Verification items for the finished model (mm, model axes). A direction names the side the tool comes from. Give positions to 0.01 mm unless a question says otherwise; leave off trailing zeros. Order: outer loops, then holes, each group sorted by start corner. A loop starts at its lowest first (then second) coordinate and runs counter-clockwise, first axis right, second up. Notation, with made-up numbers: (39.5, 17.5) - (46.5, 17.5) arc R31 ccw to (46.5, 47.5) - close; hole circle Ø3 at (25, 84). An arc over 180 degrees is marked (long way). Answer as a JSON object with one key per item and string values. Group by question number.
(1) Section check A-A (y = -3.5). Count the separate pieces of the cut face and the enclosed holes in it, then the cut area to 3 significant figures.
(2) Mould release check, pull along Z, two halves, no side actions. Record for faces 1 (the face through (6.6, 14.5, 1.156)), 2 (the face through (0, -6, -7)), 3 (the face through (0, 4, -3.844)): +Z half, -Z half, draft (parallel to the pull), parting line (faces both ways), or undercut.
(3) Thickness scan on line 1 (Z direction, x = -1.5, y = -3.5); line 2 (Z direction, x = 6.9, y = 17.5); line 3 (Y direction, x = -5.5, z = -0.5). Record the ranges inside material, lowest first.
(4) Access from +Z, -Z, +X, -X, +Y, -Y to the whole of each face (thin tool, end or side, straight path). Record for faces 4 (the face through (5, -3, -4)), 5 (the face through (-6, 0, -2)), 6 (the face through (-0.06, 3.86, -6.604)).
(5) Depth check by flat-ended pin: pin 1 Ø1 at (x, y) = (1, 5.5) entering from +Z; pin 2 Ø6 at (x, y) = (-1, 2) entering from +Z; pin 3 Ø2.5 at (x, y) = (-2, 2.5) entering from -Z. Enter the tip coordinate at first touch or a pass-through.
(6) Section check C-C (y = 3.25). Record the boundary of the cut face in (x, z), then the cut area to 3 significant figures.
```python
from build123d import *

# Parameters (mm, degrees)
SKETCH1_R                     = 8.5
BOSS_EXTRUDE1_DEPTH           = 20
BOSS_EXTRUDE1_TAPER           = 1
BOSS_EXTRUDE1_OTHER_WAY_DEPTH = 6
BOSS_EXTRUDE1_OTHER_WAY_TAPER = -1
CUT_EXTRUDE1_DEPTH            = 24.411167638
CUT_EXTRUDE1_DEPTH_BACK       = 24.411167638
CUT_EXTRUDE2_START            = -9.76024089
CUT_EXTRUDE2_OUTLINE_W        = 9.770566763
CUT_EXTRUDE2_OUTLINE_H        = 6
CUT_EXTRUDE2_DEPTH            = 9.76024089
CUT_EXTRUDE3_DEPTH            = 26.618184821
CUT_EXTRUDE3_DEPTH_BACK       = 26.618184821
SKETCH5_R                     = 1.5
FILLET1_SIZE                  = 5
CUT_EXTRUDE4_DEPTH            = 24.372877283
CUT_EXTRUDE4_DEPTH_BACK       = 24.372877283
SKETCH8_W                     = 10
SKETCH8_H                     = 6
CUT_EXTRUDE5_DEPTH            = 24.822516826
CUT_EXTRUDE6_DEPTH            = 26.618184821
CUT_EXTRUDE6_DEPTH_BACK       = 26.618184821
SKETCH9_R                     = 1.5
FILLET2_SIZE                  = 5
CUT_EXTRUDE7_DEPTH            = 29.675623685


with BuildPart() as part:
    # Sketch1 → Boss-Extrude1 (new body)
    with BuildSketch(Plane(origin=(0, 0, 0), x_dir=(1, 0, 0), z_dir=(0, 1, 0))):
        Circle(SKETCH1_R)
    extrude(amount=BOSS_EXTRUDE1_DEPTH, taper=BOSS_EXTRUDE1_TAPER)

    # Sketch1 → Boss-Extrude1 other way (add)
    with BuildSketch(Plane(origin=(0, 0, 0), x_dir=(1, 0, 0), z_dir=(0, 1, 0))):
        Circle(SKETCH1_R)
    extrude(amount=-BOSS_EXTRUDE1_OTHER_WAY_DEPTH, taper=BOSS_EXTRUDE1_OTHER_WAY_TAPER)

    # Sketch3 → Cut-Extrude1 (cut, two sides: drawn at the far end of the back side and taken through both)
    with BuildSketch(Plane(origin=(0, 0, 0), x_dir=(0, 0, -1), z_dir=(1, 0, 0)).offset(-CUT_EXTRUDE1_DEPTH_BACK)):
        Polygon((-1.155510401, -6), (-1.155510401, 0), (-11.155510401, 10), (-11.155510401, -6), align=None)
    extrude(amount=CUT_EXTRUDE1_DEPTH + CUT_EXTRUDE1_DEPTH_BACK, mode=Mode.SUBTRACT)

    # Cut-Extrude2: read off the stored shape, not the designer's step
    # Cut-Extrude2 outline → Cut-Extrude2 (cut)
    with BuildSketch(Plane.XY.offset(1.155510401).offset(CUT_EXTRUDE2_START)):
        with Locations((-9.885283382, -3)):
            Rectangle(CUT_EXTRUDE2_OUTLINE_W, CUT_EXTRUDE2_OUTLINE_H)
        with Locations((9.885283382, -3)):
            Rectangle(CUT_EXTRUDE2_OUTLINE_W, CUT_EXTRUDE2_OUTLINE_H)
    extrude(amount=CUT_EXTRUDE2_DEPTH, mode=Mode.SUBTRACT)

    # Sketch5 → Cut-Extrude3 (cut, two sides: drawn at the far end of the back side and taken through both)
    with BuildSketch(Plane.ZY.offset(5).offset(-CUT_EXTRUDE3_DEPTH_BACK)):
        with Locations(Location((-1.344489599, -3.5, 0), (0, 0, 270))):
            Circle(SKETCH5_R)
    extrude(amount=CUT_EXTRUDE3_DEPTH + CUT_EXTRUDE3_DEPTH_BACK, mode=Mode.SUBTRACT)

    # Fillet1
    # a fillet whose section is not a circle: 5 mm, written as the material it takes off along each edge
    with BuildSketch(Plane(origin=(17.5, -6, 1.155510401), x_dir=(0, 0, -1), z_dir=(-1, 0, 0))) as fillet1_piece_1:
        with BuildLine():
            Bezier((FILLET1_SIZE, 0), (0, 0), (0, -FILLET1_SIZE), weights=[1, 1.5, 1])
            Line((0, -FILLET1_SIZE), (0, 0))
            Line((0, 0), (FILLET1_SIZE, 0))
        make_face()
    extrude(amount=35, mode=Mode.SUBTRACT)

    # Sketch7 → Cut-Extrude4 (cut, two sides: drawn at the far end of the back side and taken through both)
    with BuildSketch(Plane(origin=(0, 0, 0), x_dir=(0, 0, -1), z_dir=(1, 0, 0)).offset(-CUT_EXTRUDE4_DEPTH_BACK)):
        Polygon((-1.155510401, 20), (-1.155510401, 14), (-12.24506556, 2.91044484), (-12.24506556, 20), align=None)
    extrude(amount=CUT_EXTRUDE4_DEPTH + CUT_EXTRUDE4_DEPTH_BACK, mode=Mode.SUBTRACT)

    # Sketch8 → Cut-Extrude5 (cut, through all)
    with BuildSketch(Plane.XY.offset(1.155510401)):
        with Locations((0, 17)):
            Rectangle(SKETCH8_W, SKETCH8_H)
    extrude(amount=-CUT_EXTRUDE5_DEPTH, mode=Mode.SUBTRACT)

    # Sketch9 → Cut-Extrude6 (cut, two sides: drawn at the far end of the back side and taken through both)
    with BuildSketch(Plane(origin=(-5, 0, 0), x_dir=(0, 0, -1), z_dir=(1, 0, 0)).offset(-CUT_EXTRUDE6_DEPTH_BACK)):
        with Locations(Location((1.344489599, 17.5, 0), (0, 0, 314.198748603))):
            Circle(SKETCH9_R)
    extrude(amount=CUT_EXTRUDE6_DEPTH + CUT_EXTRUDE6_DEPTH_BACK, mode=Mode.SUBTRACT)

    # Fillet2
    # a fillet whose section is not a circle: 5 mm, written as the material it takes off along each edge
    with BuildSketch(Plane(origin=(-20.568577654, 20, 1.155510401), x_dir=(0, 0, -1), z_dir=(1, 0, 0))) as fillet2_piece_1:
        with BuildLine():
            Bezier((FILLET2_SIZE, 0), (0, 0), (0, -FILLET2_SIZE), weights=[1, 1.5, 1])
            Line((0, -FILLET2_SIZE), (0, 0))
            Line((0, 0), (FILLET2_SIZE, 0))
        make_face()
    extrude(amount=28.068577654, mode=Mode.SUBTRACT)
    with BuildSketch(Plane(origin=(-7.5, 20, 1.155510401), x_dir=(0, -1, 0), z_dir=(1, 0, 0))) as fillet2_piece_2:
        with BuildLine():
            Bezier((FILLET2_SIZE, 0), (0, 0), (0, FILLET2_SIZE), weights=[1, 1.5, 1])
            Line((0, FILLET2_SIZE), (0, 0))
            Line((0, 0), (FILLET2_SIZE, 0))
        make_face()
    extrude(amount=28.068577654, mode=Mode.SUBTRACT)

    # Sketch10 → Cut-Extrude7 (cut, through all)
    with BuildSketch(Plane.XZ.offset(6)):
        with BuildLine():
            Line((-4, -3.844489599), (-4, -5.255707709))
            ThreePointArc((-4, -5.255707709), (0, -6.60473039), (4, -5.255707709))
            Line((4, -5.255707709), (4, -3.844489599))
            Line((4, -3.844489599), (-4, -3.844489599))
        make_face()
    extrude(amount=-CUT_EXTRUDE7_DEPTH, mode=Mode.SUBTRACT)


solid = part.part
```
Solutions:
{
 "1": {"separate pieces": "2", "enclosed holes": "1", "area": "41.1 mm2"},
 "2": {"face 1": "+Z half", "face 2": "draft", "face 3": "undercut"},
 "3": {"line 1": "z = -8.43 to -6.43, -3.84 to -2.84, 0.16 to 0.93", "line 2": "z = -4.42 to -2.84, 0.16 to 0.93", "line 3": "y = 0 to 16.26, 18.74 to 19.47"},
 "4": {"face 4": "+Z, -Z, +X, -Y", "face 5": "+Z, -Z, -X, -Y", "face 6": "+Y, -Y"},
 "5": {"pin 1": "stops at z = 7.16", "pin 2": "stops at z = 6.16", "pin 3": "stops at z = -8.43"},
 "6": {"outline": "(-7.2, 4.41) arc R8.44 ccw (long way) to (7.2, 4.41) - close; hole (-4, -5.26) arc R6.6 ccw to (4, -5.26) - (4, -3.84) - (-4, -3.84) - close", "area": "164 mm2"}
}
